Work out the finished part from the listing and answer in its coordinate system (mm). Face numbers are marked on the shaded views. A direction names the side the tool comes from. Coordinates: 2 decimals unless noted, no trailing zeros. Order: outer loops, then holes, each group sorted by start corner. A loop starts at its lowest first (then second) coordinate and runs counter-clockwise, first axis right, second up. Notation, with made-up numbers: (-30.5, 27) - (-10.5, 27) arc R15 cw to (-10.5, 47) - close; hole circle Ø9 at (78, -4.75). An arc over 180 degrees is marked (long way). Answer as a JSON object with one key per item and string values. Group by question number.
1) Section A-A (z = 0) is taken. Give the vertices of the cut face in (x, y), plus the area to 3 significant figures.
2) Section C-C (x = 42) is taken. Give the vertices of the cut face in (y, z), plus the area to 3 significant figures.
3) Section B-B (y = -31) is taken. Give the vertices of the cut face in (x, z), plus the area to 3 significant figures.
4) A tool of negligible diameter and unlimited length cuts with its end or side. For the marked faces 4, 5 and 6, from which of +Z, -Z, +X, -X, +Y, -Y can it reach the whole face along a straight path? Write none if from no direction.
5) Each of these flat-tipped pins is pushed along its axis until it touches: P1, Ø20, axis at x = -87.5, y = 28, coming from the -Z side; P2, Ø6, axis at x = 19, y = 9.5, coming from the +Z side; P3, Ø19, axis at x = 45, y = -27.5, coming from the -Z side. Where does it stop, or does it pass through?
6) Find the intervals of material crossed by line 1 along Y through (x, z) = (37, 0); line 2 along X through (y, z) = (18.5, 53); line 3 along X through (y, z) = (20, 37.5), in increasing order.
7) The mould has two halves that part along X. Classify the marked faces 1, 2 and 3: released by +X, released by -X, zero draft, split by the parting line, or undercut.
8) Section D-D (x = -2.5) is taken. Give the vertices of the cut face in (y, z), plus the area to 3 significant figures.
Autodesk Inventor part; units mm, degrees
ref_plane "YZ Plane" through (0, 0, 0) normal (1, 0, 0) x (0, 1, 0)
ref_plane "XZ Plane" through (0, 0, 0) normal (0, 1, 0) x (-1, 0, 0)
ref_plane "XY Plane" through (0, 0, 0) normal (0, 0, 1) x (1, 0, 0)
sketch "Sketch1" plane through (0, 0, 0) normal (0, 1, 0) x (-1, 0, 0)
  line L0 (-126.3701, 48.161) -> (-51.2671, 4.8003) construction
  line L1 (-51.2671, 4.8003) -> (-126.3701, -38.5605) construction
  line L2 (-126.3701, -38.5605) -> (-126.3701, 48.161) construction
  line L3 (110.9585, 0) -> (-59.5814, 0) construction
  line L4 (83.2089, 69.641) -> (63.2089, 35)
  line L5 (63.2089, 35) -> (-58.0347, 105)
  line L6 (-58.0347, 105) -> (-68.0347, 87.6795)
  line L7 (-68.0347, 87.6795) -> (-50.7142, 77.6795)
  line L8 (-33.3937, 67.6795) -> (40.2185, 25.1795)
  line L9 (83.2089, -69.641) -> (63.2089, -35)
  line L10 (63.2089, -35) -> (-58.0347, -105)
  line L11 (-58.0347, -105) -> (-68.0347, -87.6795)
  line L12 (-68.0347, -87.6795) -> (-50.7142, -77.6795)
  line L13 (-33.3937, -67.6795) -> (40.2185, -25.1795)
  arc A0 (83.2089, -69.641) -> (83.2089, 69.641) centre (55.3678, 0) ccw
  line L14 (-50.7142, 77.6795) -> (-50.7142, -77.6795)
  line L15 (-33.3937, 67.6795) -> (-33.3937, -67.6795)
  line L16 (40.2185, 25.1795) -> (40.2185, -25.1795)
  dimension "d3" = 40
  dimension "d4" = 140
  dimension "d5" = 20
  dimension "d7" = 20
  dimension "d19" = 70
  dimension "d20" = 75
  dimension "d21" = 20
  dimension "d22" = 85
extrude "Extrusion1" add sketch "Sketch1" along normal blind 40
sketch "Sketch2" plane through (-63.2089, 0, 35) normal (0.866, 0, 0.5) x (0.5, 0, -0.866)
  circle A0 centre (-20, 20) radius 3.4
  line L0 (-40, 40) -> (0, 40)
  line L1 (-40, 0) -> (-40, 40)
  point P0 (61.9153, 0)
  point P1 (-20, 40)
  point P2 (-40, 20)
  dimension "d10" = 6.8
extrude "Extrusion2" add sketch "Sketch2" along normal blind 10
sketch "Sketch3" plane through (-83.2089, 0, -69.641) normal (0.866, 0, -0.5) x (-0.5, 0, -0.866)
  circle A0 centre (-20, 20) radius 3.4
  line L0 (-40, 40) -> (0, 40)
  line L1 (0, 0) -> (0, 40)
  point P0 (-101.9153, 0)
  point P1 (-20, 40)
  point P2 (0, 20)
  dimension "d13" = 6.8
extrude "Extrusion3" add sketch "Sketch3" along normal blind 10
sketch "Sketch4" plane through (0, 40, 0) normal (0, 1, 0) x (1, 0, 0)
  line L0 (-105.2185, -20) -> (-65.2185, -20)
  line L1 (-65.2185, -20) -> (-65.2185, 20)
  line L2 (-65.2185, 20) -> (-105.2185, 20)
  line L3 (-105.2185, 20) -> (-105.2185, -20)
  line L4 (-40.2185, -25.1795) -> (-40.2185, 25.1795)
  point P0 (0, 0)
  point P1 (-105.2185, 0)
  dimension "d16" = 40
  dimension "d17" = 40
  dimension "d23" = 25
extrude "Extrusion4" cut sketch "Sketch4" against normal blind 40
fillet "Fillet1" radius 10 2 edges at (-40.2185, 20, -25.1795) (-40.2185, 20, 25.1795)
fillet "Fillet2" radius 13 2 edges at (33.3937, 20, 67.6795) (33.3937, 20, -67.6795)
fillet "Fillet3" radius 15 2 edges at (50.7142, 20, 77.6795) (50.7142, 20, -77.6795)
sketch "Sketch5" plane through (68.0347, 0, 87.6795) normal (0.5, 0, -0.866) x (-0.866, 0, -0.5)
  point P0 (102.7595, 0)
  point P1 (5.815, 19.918)
hole "Hole1" at (62.9988, 19.918, 84.772) direction (-0.5, 0, 0.866) diameter 4 end through all counterbore diameter 5 counterbore depth 2
sketch "Sketch6" plane through (-35.2185, 0, 28.0662) normal (0.5, 0, -0.866) x (-0.866, 0, -0.5)
  point P0 (-16.467, 0)
  point P1 (-7.7378, 18.9937)
hole "Hole2" at (-28.5174, 18.9937, 31.9351) direction (-0.5, 0, 0.866) diameter 4 end through all counterbore diameter 5 counterbore depth 2
fillet "Fillet9" radius 1 2 edges at (-130.3678, 0, 0) (-130.3678, 40, 0)
sketch "Sketch11" plane through (0, 0, 0) normal (0, -1, 0) x (1, 0, 0)
  line L0 (33.3937, -30) -> (50.7142, -30)
  line L1 (50.7142, -30) -> (50.7142, 30)
  line L2 (50.7142, 30) -> (33.3937, 30)
  line L3 (33.3937, 30) -> (33.3937, -30)
  line L4 (33.3937, 45.1628) -> (33.3937, -45.1628)
  line L5 (50.7142, 69.0192) -> (50.7142, -69.0192)
  point P0 (0, 0)
  point P1 (33.3937, 0)
  dimension "d89" = 60
extrude "Extrusion8" add sketch "Sketch11" along normal blind 55
sketch "Sketch12" plane through (33.3937, 0, -45.1628) normal (-1, 0, 0) x (0, 0, 1)
  circle A0 centre (45.1628, -31) radius 10
  point P0 (45.1628, 0)
  dimension "d92" = 20
  dimension "d93" = 31
extrude "Extrusion9" cut sketch "Sketch12" against normal up to next
fillet "Fillet10" radius 15 4 edges at (42.0539, 0, 30) (42.0539, -55, 30) (42.0539, 0, -30) (42.0539, -55, -30)
sketch "Sketch13" plane through (50.7142, 0, -69.0192) normal (1, 0, 0) x (0, 0, -1)
  circle A0 centre (-69.0192, 20) radius 7.5
  line L0 (-49.6132, 0) -> (-88.4252, 0)
  point P0 (-69.0192, 0)
  dimension "d97" = 15
  dimension "d98" = 20
extrude "Extrusion10" cut sketch "Sketch13" against normal up to next
properties part number "Profil_Winkel_oben"
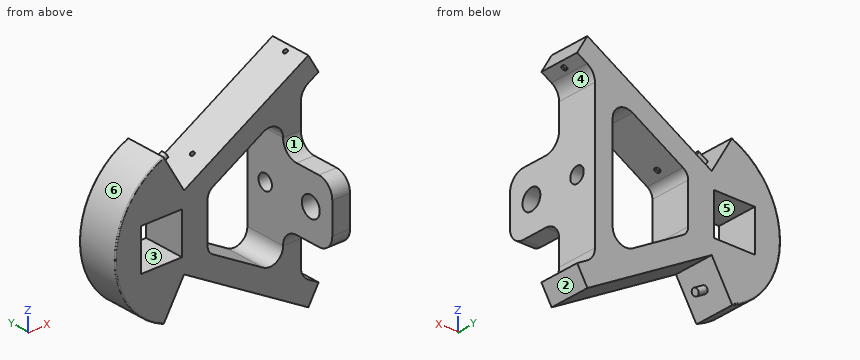
Report:
{
 "1": {"outline": "(-130.37, 1) arc R1 ccw to (-129.37, 0) - (-105.22, 0) - (-105.22, 40) - (-129.37, 40) arc R1 ccw to (-130.37, 39) - close; (-65.22, 0) - (-40.22, 0) - (-40.22, 40) - (-65.22, 40) - close; (33.39, -55) - (50.71, -55) - (50.71, -41) - (33.39, -41) - close; (33.39, -21) - (50.71, -21) - (50.71, 12.5) - (33.39, 12.5) - close; (33.39, 27.5) - (50.71, 27.5) - (50.71, 40) - (33.39, 40) - close", "area": "3,040 mm²"},
 "2": {"outline": "(-55, -15) arc R15 ccw to (-40, -30) - (-15, -30) arc R15 cw to (0, -45) - (0, -95.74) - (40, -95.74) - (40, 95.74) - (0, 95.74) - (0, 45) arc R15 cw to (-15, 30) - (-40, 30) arc R15 ccw to (-55, 15) - close; hole circle Ø20 at (-31, 0); hole circle Ø15 at (20, 0)", "area": "10,500 mm²"},
 "3": {"outline": "(33.39, -30) - (50.71, -30) - (50.71, -10) - (33.39, -10) - close; (33.39, 10) - (50.71, 10) - (50.71, 30) - (33.39, 30) - close", "area": "693 mm²"},
 "4": {"face 4": "+X, +Y, -Y", "face 5": "+Y, -Y", "face 6": "-X, +Y, -Y"},
 "5": {"P1": "stops at z = -69.64", "P2": "stops at z = 84.2", "P3": "stops at z = -30"},
 "6": {"line 1": "y = -55 to -41, -21 to 12.5, 27.5 to 40", "line 2": "x = -108.43 to -65.93, -32.03 to 7.97, 30.77 to 50.71", "line 3": "x = -120.32 to -64.65, -58.88 to -33.73, -29.73 to -18.88, 33.39 to 50.71"},
 "7": {"face 1": "zero draft", "face 2": "released by +X", "face 3": "undercut"},
 "8": {"outline": "(0, -70.05) - (40, -70.05) - (40, -46.96) - (0, -46.96) - close; (0, 46.96) - (40, 46.96) - (40, 70.05) - (0, 70.05) - close", "area": "1,850 mm²"}
}
